```python
from build123d import *

# Parameters (mm, degrees)
BOSS_EXTRUDE1_DEPTH = 6
SKETCH3_W           = 53.5
SKETCH3_H           = 30
BOSS_EXTRUDE2_DEPTH = 30
SKETCH4_W           = 34.5
SKETCH4_H           = 4.75
CUT_EXTRUDE1_DEPTH  = 240


with BuildPart() as part:
    # Sketch2 → Boss-Extrude1 (new body)
    with BuildSketch(Plane(origin=(0, 0, 0), x_dir=(1, 0, 0), z_dir=(0, 1, 0))):
        with BuildLine():
            Line((10, 0), (67.5, 0))
            ThreePointArc((67.5, 0), (74.571067812, 2.928932188), (77.5, 10))
            Line((77.5, 10), (77.5, 254))
            ThreePointArc((77.5, 254), (74.571067812, 261.071067812), (67.5, 264))
            Line((67.5, 264), (10, 264))
            ThreePointArc((10, 264), (2.928932188, 261.071067812), (0, 254))
            Line((0, 254), (0, 10))
            ThreePointArc((0, 10), (2.928932188, 2.928932188), (10, 0))
        make_face()
    extrude(amount=BOSS_EXTRUDE1_DEPTH)

    # Sketch3 → Boss-Extrude2 (add)
    with BuildSketch(Plane(origin=(0, 6, 0), x_dir=(1, 0, 0), z_dir=(0, 1, 0))):
        with Locations((38.75, 27)):
            Rectangle(SKETCH3_W, SKETCH3_H)
        with Locations((38.75, 69)):
            Rectangle(SKETCH3_W, SKETCH3_H)
        with Locations((38.75, 111)):
            Rectangle(SKETCH3_W, SKETCH3_H)
        with Locations((38.75, 237)):
            Rectangle(SKETCH3_W, SKETCH3_H)
        with Locations((38.75, 195)):
            Rectangle(SKETCH3_W, SKETCH3_H)
        with Locations((38.75, 153)):
            Rectangle(SKETCH3_W, SKETCH3_H)
    extrude(amount=BOSS_EXTRUDE2_DEPTH)

    # Sketch4 → Cut-Extrude1 (cut)
    with BuildSketch(Plane.XY.offset(-12)):
        with BuildLine():
            Line((21.5, 36), (16.75, 36))
            ThreePointArc((16.75, 36), (20.108757211, 34.608757211), (21.5, 31.25))
            Line((21.5, 31.25), (21.5, 36))
        make_face()
        with Locations((38.75, 33.625)):
            Rectangle(SKETCH4_W, SKETCH4_H)
        with BuildLine():
            Line((56, 36), (56, 31.25))
            ThreePointArc((56, 31.25), (57.391242789, 34.608757211), (60.75, 36))
            Line((60.75, 36), (56, 36))
        make_face()
        with BuildLine():
            Line((65.5, 36), (60.75, 36))
            ThreePointArc((60.75, 36), (64.108757211, 34.608757211), (65.5, 31.25))
            Line((65.5, 31.25), (65.5, 36))
        make_face()
        with BuildLine():
            Line((12, 36), (16.75, 36))
            ThreePointArc((16.75, 36), (13.391242789, 34.608757211), (12, 31.25))
            Line((12, 31.25), (12, 36))
        make_face()
    extrude(amount=-CUT_EXTRUDE1_DEPTH, mode=Mode.SUBTRACT)


solid = part.part
```
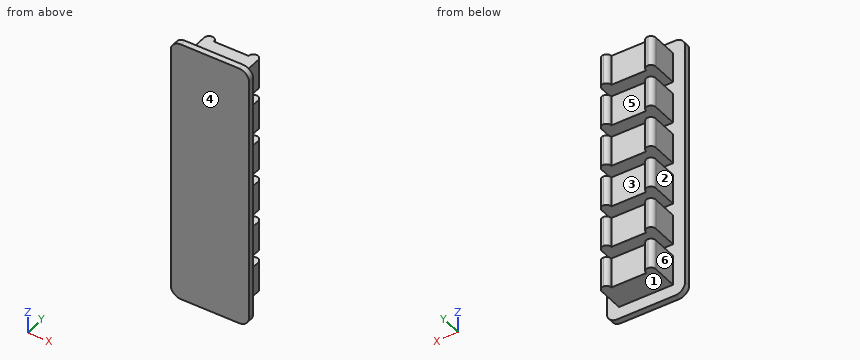
Check sheet for the modelled part. Datum: model origin and axes. Units: mm. Face numbers are marked on the shaded views. A direction names the side the tool comes from. Give positions to 0.01 mm unless a question says otherwise; leave off trailing zeros. Order: outer loops, then holes, each group sorted by start corner. A loop starts at its lowest first (then second) coordinate and runs counter-clockwise, first axis right, second up. Notation, with made-up numbers: M 58,10.5 L 70,10.5 A22 ccw 70,20.5 Z; hole C 41.5,0 d10. An arc over 180 degrees is marked long. Answer in a Markdown table with one row per item. Add a question column.
Q1. Sectioned sample at D-D, the plane y = 33.5. Count the separate pieces of the cut face and the enclosed holes in it, and give its area (3 significant figures).
Q2. Thickness scan on L1, parallel to Z at x = 32.5, y = 27.5; L2, parallel to Y at x = 25.5, z = -91.5; L3, parallel to Y at x = 24.5, z = -158. Record the ranges inside material, lowest first.
Q3. Access from +Z, -Z, +X, -X, +Y, -Y to the whole of each face (thin tool, end or side, straight path). Record for the marked faces 4, 5 and 6.
Q4. Sectioned sample at C-C, the plane z = -200. Record the boundary of the cut face in (x, y), and give its area (3 significant figures).
Q5. Gauge pin test, flat ends, axial feed: pin 1 Ø8 at (x, z) = (9.5, -116.5) entering from +Y; pin 2 Ø7.5 at (y, z) = (13, -244.5) entering from -X; pin 3 Ø3 at (x, z) = (36.5, -73.5) entering from +Y; pin 4 Ø10 at (x, y) = (23, 8.5) entering from +Z. Record the tip position at first contact, or that the pin passes through.
Q6. Sectioned sample at B-B, the plane x = 46. Record the boundary of the cut face in (y, z), and give its area (3 significant figures).
Q7. Release check for a two-part mould opening along X. For the marked faces 1, 2 and 3 record: released by +X, released by -X, zero draft, split by the parting line, or undercut.
Q8. Sectioned sample at A-A, the plane y = 22.5. Record the boundary of the cut face in (x, z), and give its area (3 significant figures).
Verdict:
| question | item | result |
|---|---|---|
| 1 | separate pieces | 12 |
| 1 | enclosed holes | 0 |
| 1 | area | 3,010 mm² |
| 2 | L1 | -252 to -222, -210 to -180, -168 to -138, -126 to -96, -84 to -54, -42 to -12 |
| 2 | L2 | 0 to 6 |
| 2 | L3 | 0 to 31.25 |
| 3 | face 4 | +Z, -Z, +X, -X, -Y |
| 3 | face 5 | +Z, -Z, +Y |
| 3 | face 6 | +Z, -Z, -X, +Y |
| 4 | outline | M 0,0 L 77.5,0 L 77.5,6 L 65.5,6 L 65.5,31.25 A4.75 ccw 56,31.25 L 21.5,31.25 A4.75 ccw 12,31.25 L 12,6 L 0,6 Z |
| 4 | area | 1,890 mm² |
| 5 | pin 1 | y = 34.71 |
| 5 | pin 2 | x = 12 |
| 5 | pin 3 | y = 31.25 |
| 5 | pin 4 | z = 0 |
| 6 | outline | M 0,-264 L 6,-264 L 6,-252 L 31.25,-252 L 31.25,-222 L 6,-222 L 6,-210 L 31.25,-210 L 31.25,-180 L 6,-180 L 6,-168 L 31.25,-168 L 31.25,-138 L 6,-138 L 6,-126 L 31.25,-126 L 31.25,-96 L 6,-96 L 6,-84 L 31.25,-84 L 31.25,-54 L 6,-54 L 6,-42 L 31.25,-42 L 31.25,-12 L 6,-12 L 6,0 L 0,0 Z |
| 6 | area | 6,130 mm² |
| 7 | face 1 | zero draft |
| 7 | face 2 | released by -X |
| 7 | face 3 | undercut |
| 8 | outline | M 12,-252 L 65.5,-252 L 65.5,-222 L 12,-222 Z; M 12,-210 L 65.5,-210 L 65.5,-180 L 12,-180 Z; M 12,-168 L 65.5,-168 L 65.5,-138 L 12,-138 Z; M 12,-126 L 65.5,-126 L 65.5,-96 L 12,-96 Z; M 12,-84 L 65.5,-84 L 65.5,-54 L 12,-54 Z; M 12,-42 L 65.5,-42 L 65.5,-12 L 12,-12 Z |
| 8 | area | 9,630 mm² |
